Check sheet for the modelled part. Datum: model origin and axes. Units: mm. Face numbers are marked on the shaded views. A direction names the side the tool comes from. Round coordinates to 2 decimals unless told otherwise and drop trailing zeros. Order: outer loops, then holes, each group sorted by start corner. A loop starts at its lowest first (then second) coordinate and runs counter-clockwise, first axis right, second up.
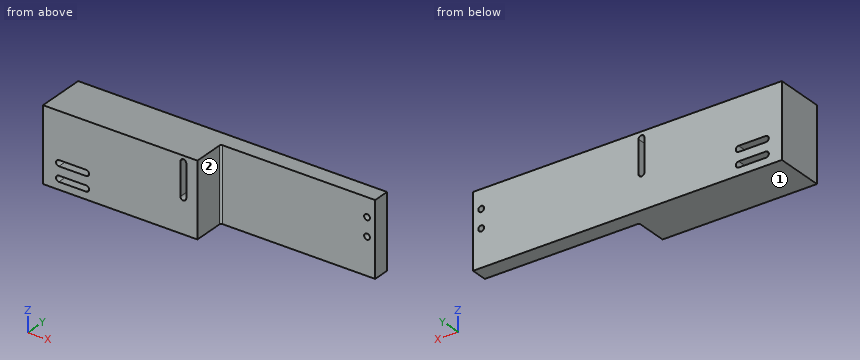
```python
from build123d import *

# Parameters (mm, degrees)
SKETCH1_W           = 170
SKETCH1_H           = 40.5
BOSS_EXTRUDE1_DEPTH = 9
SKETCH2_W           = 85
SKETCH2_H           = 40.5
BOSS_EXTRUDE2_DEPTH = 17.745
SKETCH3_R           = 1.6
CUT_EXTRUDE1_DEPTH  = 92.380290681
FILLET1_R           = 1


with BuildPart() as part:
    # Sketch1 → Boss-Extrude1 (new body)
    with BuildSketch(Plane(origin=(0, 0, 0), x_dir=(1, 0, 0), z_dir=(0, 1, 0))):
        Rectangle(SKETCH1_W, SKETCH1_H)
    extrude(amount=BOSS_EXTRUDE1_DEPTH)

    # Sketch2 → Boss-Extrude2 (add)
    with BuildSketch(Plane.XZ):
        with Locations((-42.5, 0)):
            Rectangle(SKETCH2_W, SKETCH2_H)
    extrude(amount=BOSS_EXTRUDE2_DEPTH)

    # Sketch3 → Cut-Extrude1 (cut, through all)
    with BuildSketch(Plane(origin=(0, 9, 0), x_dir=(1, 0, 0), z_dir=(0, 1, 0))):
        with Locations(Location((80.508679868, 0, 0), (0, 0, 270))):
            Circle(SKETCH3_R)
        with Locations(Location((80.508679868, -10, 0), (0, 0, 270))):
            Circle(SKETCH3_R)
        with BuildLine():
            Line((-76.241320132, 8.185093605), (-61.241320132, 8.185093605))
            ThreePointArc((-61.241320132, 8.185093605), (-59.641320132, 6.585093605), (-61.241320132, 4.985093605))
            Line((-61.241320132, 4.985093605), (-76.241320132, 4.985093605))
            ThreePointArc((-76.241320132, 4.985093605), (-77.841320132, 6.585093605), (-76.241320132, 8.185093605))
        make_face()
        with BuildLine():
            Line((-61.241320132, 12.985093605), (-76.241320132, 12.985093605))
            ThreePointArc((-76.241320132, 12.985093605), (-77.841320132, 14.585093605), (-76.241320132, 16.185093605))
            Line((-76.241320132, 16.185093605), (-61.241320132, 16.185093605))
            ThreePointArc((-61.241320132, 16.185093605), (-59.641320132, 14.585093605), (-61.241320132, 12.985093605))
        make_face()
        with BuildLine():
            Line((-6.141320132, 1.249202664), (-6.141320132, -16.750797336))
            ThreePointArc((-6.141320132, -16.750797336), (-7.741320132, -18.350797336), (-9.341320132, -16.750797336))
            Line((-9.341320132, -16.750797336), (-9.341320132, 1.249202664))
            ThreePointArc((-9.341320132, 1.249202664), (-7.741320132, 2.849202664), (-6.141320132, 1.249202664))
        make_face()
    extrude(amount=-CUT_EXTRUDE1_DEPTH, mode=Mode.SUBTRACT)

    # Fillet1
    fillet1_edges = [part.edges().sort_by_distance(p)[0] for p in [
        (0, 0, 0),
    ]]
    fillet(fillet1_edges, radius=FILLET1_R)


solid = part.part
```
Item 1: Go/stop test with flat-tipped pins: P1, Ø5, axis at y = -12.5, z = 2, coming from the +X side; P2, Ø3.5, axis at x = 80.51, z = 0, coming from the -Y side. Record where each tip stops, or that it passes through.
Answer:
P1: stops at x = 0
P2: stops at y = 0
Item 2: Sectioned sample at B-B (y = -14.75). Record the cut outline in (x, z), and give its area (3 significant figures).
Answer:
outline: (-85, -20.25) - (0, -20.25) - (0, 20.25) - (-85, 20.25) - close; hole (-76.24, -16.19) - (-61.24, -16.19) arc R1.6 ccw to (-61.24, -12.99) - (-76.24, -12.99) arc R1.6 ccw to start; hole (-76.24, -8.19) - (-61.24, -8.19) arc R1.6 ccw to (-61.24, -4.99) - (-76.24, -4.99) arc R1.6 ccw to start; hole (-9.34, -1.25) arc R1.6 ccw to (-6.14, -1.25) - (-6.14, 16.75) arc R1.6 ccw to (-9.34, 16.75) - close
area: 3,260 mm2
Item 3: Scan lines: line 1 along X through (y, z) = (2, 10); line 2 along X through (y, z) = (4.5, 10.5); line 3 along X through (y, z) = (-4.75, 16). Record each from-to range of solid material in increasing order.
Answer:
line 1: x = -85 to -9.34, -6.14 to 78.91, 82.11 to 85
line 2: x = -85 to -9.34, -6.14 to 78.99, 82.03 to 85
line 3: x = -85 to -9.34, -6.14 to 0
Item 4: Access from +Z, -Z, +X, -X, +Y, -Y to the whole of each face (thin tool, end or side, straight path). Record for the marked faces 1 and 2.
Answer:
face 1: -Z, +X, -X, +Y, -Y
face 2: +Z, -Z, +X, -Y
Item 5: Sectioned sample at D-D (x = 25.5). Record the cut outline in (y, z).
Answer:
outline: (0, -20.25) - (9, -20.25) - (9, 20.25) - (0, 20.25) - close
Item 6: Sectioned sample at A-A (z = 10). Record the cut outline in (x, y) (3 decimals).
Answer:
outline: (-85, -17.745) - (-9.341, -17.745) - (-9.341, 9) - (-85, 9) - close; (-6.141, -17.745) - (0, -17.745) - (0, -1) arc R1 cw to (1, 0) - (78.909, 0) - (78.909, 9) - (-6.141, 9) - close; (82.109, 0) - (85, 0) - (85, 9) - (82.109, 9) - close
Item 7: Sectioned sample at C-C (y = 6.25). Record the cut outline in (x, z).
Answer:
outline: (-85, -20.25) - (85, -20.25) - (85, 20.25) - (-85, 20.25) - close; hole (-76.24, -16.19) - (-61.24, -16.19) arc R1.6 ccw to (-61.24, -12.99) - (-76.24, -12.99) arc R1.6 ccw to start; hole (-76.24, -8.19) - (-61.24, -8.19) arc R1.6 ccw to (-61.24, -4.99) - (-76.24, -4.99) arc R1.6 ccw to start; hole (-9.34, -1.25) arc R1.6 ccw to (-6.14, -1.25) - (-6.14, 16.75) arc R1.6 ccw to (-9.34, 16.75) - close; hole circle Ø3.2 at (80.51, 0); hole circle Ø3.2 at (80.51, 10)
